from build123d import *

# Parameters (mm, degrees)
SKETCH1_R               = 10
BOSS_EXTRUDE1_DEPTH     = 191.5
SKETCH2_R               = 8.5
BOSS_EXTRUDE2_DEPTH     = 103
SKETCH4_R               = 8.5
BOSS_EXTRUDE3_DEPTH     = 67.5
FILLET1_R               = 0.5
FILLET2_R               = 0.5
SKETCH6_R               = 7.5
BOSS_EXTRUDE4_DEPTH     = 20
CUT_EXTRUDE1_DEPTH      = 1.8
SKETCH8_R               = 17.075
SKETCH8_R_2             = 7.075
CUT_EXTRUDE_THIN1_DEPTH = 1
FILLET3_R               = 0.25
CHAMFER1_SIZE           = 1
CHAMFER2_SIZE           = 0.5


with BuildPart() as part:
    # Sketch1 → Boss-Extrude1 (new body)
    with BuildSketch(Plane.XY):
        Circle(SKETCH1_R)
    extrude(amount=BOSS_EXTRUDE1_DEPTH)

    # Sketch2 → Boss-Extrude2 (add)
    with BuildSketch(Plane.XY.offset(191.5)):
        Circle(SKETCH2_R)
    extrude(amount=BOSS_EXTRUDE2_DEPTH)

    # Sketch4 → Boss-Extrude3 (add)
    with BuildSketch(Plane(origin=(0, 0, 0), x_dir=(-1, 0, 0), z_dir=(0, 0, -1))):
        Circle(SKETCH4_R)
    extrude(amount=BOSS_EXTRUDE3_DEPTH)

    # Fillet1
    fillet1_edges = [part.edges().sort_by_distance(p)[0] for p in [
        (-10, 0, 191.5),
    ]]
    fillet(fillet1_edges, radius=FILLET1_R)

    # Fillet2
    fillet2_edges = [part.edges().sort_by_distance(p)[0] for p in [
        (-10, 0, 0),
    ]]
    fillet(fillet2_edges, radius=FILLET2_R)

    # Sketch6 → Boss-Extrude4 (add)
    with BuildSketch(Plane(origin=(0, 0, -67.5), x_dir=(-1, 0, 0), z_dir=(0, 0, -1))):
        Circle(SKETCH6_R)
    extrude(amount=BOSS_EXTRUDE4_DEPTH)

    # Sketch7 → Cut-Extrude1 (cut)
    with BuildSketch(Plane(origin=(0, 7.5, 0), x_dir=(-1, 0, 0), z_dir=(0, 1, 0))):
        with BuildLine():
            Line((2.25, -75.5), (2.25, -71.5))
            ThreePointArc((2.25, -71.5), (0, -69.25), (-2.25, -71.5))
            Line((-2.25, -71.5), (-2.25, -75.5))
            ThreePointArc((-2.25, -75.5), (0, -77.75), (2.25, -75.5))
        make_face()
    extrude(amount=-CUT_EXTRUDE1_DEPTH, mode=Mode.SUBTRACT)

    # Sketch8 → Cut-Extrude-Thin1 (cut)
    with BuildSketch(Plane.XY.offset(-83.5)):
        Circle(SKETCH8_R)
        Circle(SKETCH8_R_2, mode=Mode.SUBTRACT)
    extrude(amount=-CUT_EXTRUDE_THIN1_DEPTH, mode=Mode.SUBTRACT)

    # Fillet3
    fillet3_edges = [part.edges().sort_by_distance(p)[0] for p in [
        (8.5, 0, -67.5),
    ]]
    fillet(fillet3_edges, radius=FILLET3_R)

    # Chamfer1
    chamfer1_edges = [part.edges().sort_by_distance(p)[0] for p in [
        (7.5, 0, -87.5),
    ]]
    chamfer(chamfer1_edges, length=CHAMFER1_SIZE)

    # Chamfer2
    chamfer2_edges = [part.edges().sort_by_distance(p)[0] for p in [
        (-8.5, 0, 294.5),
    ]]
    chamfer(chamfer2_edges, length=CHAMFER2_SIZE)


solid = part.part
Work out the finished part from the listing and answer in its coordinate system (mm). A direction names the side the tool comes from. Round coordinates to 2 decimals unless told otherwise and drop trailing zeros. Write each loop counter-clockwise with the first axis right and the second up, starting at its lowest first coordinate (ties: lowest second). Pieces come first, ordered by that corner, then holes. Notation, with made-up numbers: (87, 67) - (101, 67) arc R21 ccw to (101, 98) - close; hole circle Ø3 at (-13, 13.25). An arc over 180 degrees is marked (long way). Answer in a Markdown table with one row per item. Add a question column.
1. For faces 1 (the cylindrical face through (-4.57, 7.167, -33.154)), 2 (the cylindrical face through (3.26, -6.28, -83.99)), 3 (the flat face through (0, 0, -87.5)), 4 (the flat face through (-2.2, -8.4, 191.5)), determine the directions among +Z, -Z, +X, -X, +Y, -Y from which every point of the face is accessible in a straight line to the end or side of a thin tool.
2. Find the intervals of material crossed by line 1 along X through (y, z) = (1, 111); line 2 along Z through (x, y) = (-2.5, 7.5); line 3 along Y through (x, z) = (0.25, 112), in increasing order. Write a range as from..to.
3. The mould has two halves that part along Z. Classify faces 5 (the flat face through (3.9, -6.1, -83.5)), 6 (the cylindrical face through (-2.17, -9.76, 94.42)), 7 (the flat face through (-4, -7, -67.5)), 8 (the flat face through (0, 0, 294.5)): +Z half, -Z half, draft (parallel to the pull), parting line (faces both ways), or undercut.
4. A cutting plane is placed at B-B, the plane z = 22. Determine the outline of the cut face in (x, y), and give its area (3 significant figures).
5. Given pin 1 (5 mm diameter, centred on x = 1, z = -75.5, fed in from +Y); pin 2 (1.6 mm diameter, centred on y = 6.5, z = -73.5, fed in from -X); pin 3 (1 mm diameter, centred on y = 2, z = -9, fed in from +X), each flat-ended and moving along its own axis, determine where each tip first touches the part or whether it passes through.
6. A cutting plane is placed at C-C, the plane z = 211. Determine the outline of the cut face in (x, y), and give its area (3 significant figures).
Worked out:
| question | item | result |
|---|---|---|
| 1 | face 1 | -Z |
| 1 | face 2 | none |
| 1 | face 3 | -Z, +X, -X, +Y, -Y |
| 1 | face 4 | +Z |
| 2 | line 1 | -9.95..9.95 |
| 2 | line 2 | -67.5..294.5 |
| 2 | line 3 | -10..10 |
| 3 | face 5 | undercut |
| 3 | face 6 | draft |
| 3 | face 7 | -Z half |
| 3 | face 8 | +Z half |
| 4 | outline | circle Ø20 at (0, 0) |
| 4 | area | 314 mm^2 |
| 5 | pin 1 | y = 7.5 |
| 5 | pin 2 | x = -4.87 |
| 5 | pin 3 | x = 8.37 |
| 6 | outline | circle Ø17 at (0, 0) |
| 6 | area | 227 mm^2 |
